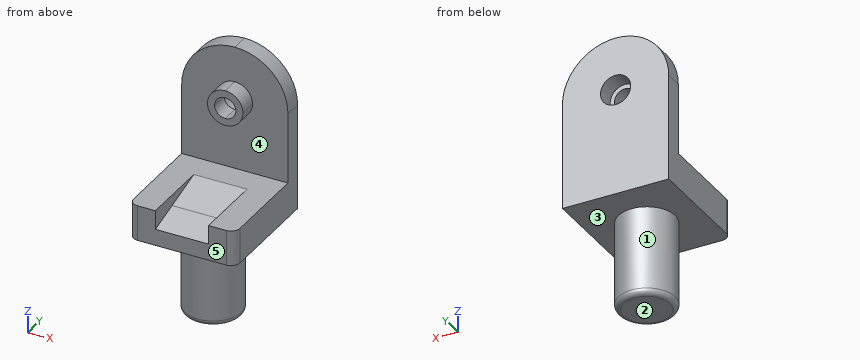
from build123d import *

# Parameters (mm, degrees)
F0_R      = 16
F1_DEPTH  = 50
F3_DEPTH  = 20
F4_DEPTH  = 20
F6_DEPTH  = 30
F7_DEPTH  = 40
F8_W      = 60
F8_H      = 10
F9_DEPTH  = 70
F10_R     = 29.99999
F11_R     = 3
F12_R     = 5
F14_D     = 17
F15_DEPTH = 10


# Not quite as in the source:
# - a fillet or chamfer is up to 0.001 mm smaller than in the source, because OpenCascade refuses the exact size


with BuildPart() as f1:
    # F0 (on Top) → F1 (new body)
    with BuildSketch(Plane.XY):
        Circle(F0_R)
    extrude(amount=F1_DEPTH)

    # F2 (on face) → F3 (join)
    with BuildSketch(Plane.XY.offset(50)):
        with BuildLine():
            Line((-30, 32.5), (-30, 7.5))
            Line((-30, 7.5), (-14.1332940251, 7.5))
            ThreePointArc((-14.1332940251, 7.5), (0, 16), (14.1332940251, 7.5))
            Line((14.1332940251, 7.5), (15, 7.5))
            Line((15, 7.5), (30, 7.5))
            Line((30, 7.5), (30, 32.5))
            Line((30, 32.5), (0, 32.5))
            Line((0, 32.5), (-30, 32.5))
        make_face()
        with BuildLine():
            ThreePointArc((14.1332940251, 7.5), (0, 16), (-14.1332940251, 7.5))
            Line((-14.1332940251, 7.5), (14.1332940251, 7.5))
        make_face()
    extrude(amount=F3_DEPTH)

    # F2 (on face) → F4 (join)
    with BuildSketch(Plane.XY.offset(50)):
        with BuildLine():
            Line((15, 5.5677643628), (15, -5.5677643628))
            ThreePointArc((15, -5.5677643628), (15.748015748, -2.8284271247), (16, 0))
            ThreePointArc((16, 0), (15.748015748, 2.8284271247), (15, 5.5677643628))
        make_face()
        with BuildLine():
            ThreePointArc((16, 0), (15.748015748, -2.8284271247), (15, -5.5677643628))
            Line((15, -5.5677643628), (15, -32.5))
            Line((15, -32.5), (30, -32.5))
            Line((30, -32.5), (30, 0))
            Line((30, 0), (30, 7.5))
            Line((30, 7.5), (15, 7.5))
            Line((15, 7.5), (15, 5.5677643628))
            ThreePointArc((15, 5.5677643628), (15.748015748, 2.8284271247), (16, 0))
        make_face()
    extrude(amount=F4_DEPTH)

    # F5 (on face) → F6 (join)
    with BuildSketch(Plane(origin=(15, 0, 0), x_dir=(0, -1, 0), z_dir=(-1, 0, 0))):
        Polygon((3.8423609018, 66.9608235561), (-7.5, 70), (-7.5, 50), (-5.5677643628, 50), (5.5677643628, 50), (32.5, 50), (32.5, 59.2820323028), (15.1847218036, 63.9216471122), align=None)
    extrude(amount=F6_DEPTH)

    # F7 (add): a face of the model
    f7_faces = [f1.faces().sort_by_distance(p)[0] for p in [
        (-22.5, 7.5, 60),
    ]]
    extrude(f7_faces, amount=F7_DEPTH)

    # F8 (on face) → F9 (join)
    with BuildSketch(Plane.XY.offset(70)):
        with Locations((0, 27.5)):
            Rectangle(F8_W, F8_H)
    extrude(amount=F9_DEPTH)

    # F10 (radius 30 in the source; OpenCascade refuses exactly that, so slightly less here)
    f10_edges = [f1.edges().sort_by_distance(p)[0] for p in [
        (-30, 27.5, 140),
        (30, 27.5, 140),
    ]]
    fillet(f10_edges, radius=F10_R)

    # F11
    f11_edges = [f1.edges().sort_by_distance(p)[0] for p in [
        (-16, 0, 0),
    ]]
    fillet(f11_edges, radius=F11_R)

    # F12
    f12_edges = [f1.edges().sort_by_distance(p)[0] for p in [
        (-30, -32.5, 60),
        (30, -32.5, 60),
    ]]
    fillet(f12_edges, radius=F12_R)

    # F14 (through all)
    with Locations(Plane.XZ.offset(-22.5)):
        with Locations((0, 110)):
            Hole(F14_D / 2)

    # F13 (on face) → F15 (join)
    with BuildSketch(Plane.XZ.offset(-22.5)):
        with BuildLine():
            Line((-6, 110), (-10, 110))
            ThreePointArc((-10, 110), (-7.0710678119, 102.9289321881), (0, 100))
            Line((0, 100), (0, 104))
            ThreePointArc((0, 104), (-4.2426406871, 105.7573593129), (-6, 110))
        make_face()
        with BuildLine():
            Line((0, 116), (0, 120))
            ThreePointArc((0, 120), (-7.0710678119, 117.0710678119), (-10, 110))
            Line((-10, 110), (-6, 110))
            ThreePointArc((-6, 110), (-4.2426406871, 114.2426406871), (0, 116))
        make_face()
        with BuildLine():
            ThreePointArc((10, 110), (7.0710678119, 117.0710678119), (0, 120))
            Line((0, 120), (0, 116))
            ThreePointArc((0, 116), (4.2426406871, 114.2426406871), (6, 110))
            Line((6, 110), (10, 110))
        make_face()
        with BuildLine():
            ThreePointArc((0, 100), (7.0710678119, 102.9289321881), (10, 110))
            Line((10, 110), (6, 110))
            ThreePointArc((6, 110), (4.2426406871, 105.7573593129), (0, 104))
            Line((0, 104), (0, 100))
        make_face()
    extrude(amount=F15_DEPTH)


solid = f1.part
Input: part model. Units: mm. Frame: model coordinates. Face numbers are marked on the shaded views. A direction names the side the tool comes from. Round coordinates to 2 decimals unless told otherwise and drop trailing zeros. Loops run counter-clockwise (first coordinate to the right, second up) from the corner with the lowest first, then second, coordinate; pieces in that order, holes last. Notation, with made-up numbers: (72, -31.75) -> (83, -31.75) arc R19 cw to (83, -20.75) -> close; hole circle Ø5 at (20.5, -0.5). An arc over 180 degrees is marked (long way). Answer as a JSON object with one key per item and string values. Group by question number.
1) Pin query (flat end, axial travel): pin 1 (13.5 mm diameter, centred on x = -0.5, z = 111.5, fed in from +Y); pin 2 (22 mm diameter, centred on x = 0, z = 110, fed in from +Y); pin 3 (12 mm diameter, centred on x = 6, z = 114.5, fed in from -Y); pin 4 (3 mm diameter, centred on x = 14, y = 8.5, fed in from -Z). Return the tip coordinate at first contact, or that it passes through.
2) Ray query, L1, parallel to Z at x = 0.5, y = 29; L2, parallel to Y at x = -15, z = 108; L3, parallel to Z at x = 19.5, y = 3.5. Return the intervals inside material, ascending.
3) Section query B-B on y = 14.5. State how many separate pieces and enclosed holes the cut face has, plus the area to 3 significant figures.
4) Section query D-D on y = 0. Output: boundary loops of the cut face in (x, z).
5) Section query C-C on x = -20.5. Output: boundary loops of the cut face in (y, z).
6) Reachability of the marked faces 1 and 2 from +Z, -Z, +X, -X, +Y, -Y: full face, straight path, thin tool, end or side. Return the list, or none.
7) Section query A-A on z = 106.5. Output: boundary loops of the cut face in (x, y), plus the area to 3 significant figures.
8) Draft query along Z for the marked faces 3, 4 and 5. Return one class per face: +Z half, -Z half, draft (parallel to the pull), parting line (faces both ways), or undercut.
Reply:
{
 "1": {"pin 1": "stops at y = 22.5", "pin 2": "stops at y = 32.5", "pin 3": "stops at y = 12.5", "pin 4": "stops at z = 0.66"},
 "2": {"L1": "z = 50 to 101.51, 118.49 to 140", "L2": "y = 22.5 to 32.5", "L3": "z = 50 to 70"},
 "3": {"separate pieces": "2", "enclosed holes": "1", "area": "2,070 mm2"},
 "4": {"outline": "(-30, 50) -> (-16, 50) -> (-16, 3) arc R3 ccw to (-13, 0) -> (13, 0) arc R3 ccw to (16, 3) -> (16, 50) -> (30, 50) -> (30, 70) -> (15, 70) -> (15, 67.99) -> (-15, 67.99) -> (-15, 70) -> (-30, 70) -> close"},
 "5": {"outline": "(-32.5, 50) -> (32.5, 50) -> (32.5, 131.9) -> (22.5, 131.9) -> (22.5, 70) -> (-32.5, 70) -> close"},
 "6": {"face 1": "-Z", "face 2": "-Z, +X, -X, +Y, -Y"},
 "7": {"outline": "(-30, 22.5) -> (-9.37, 22.5) -> (-9.37, 12.5) -> (-4.87, 12.5) -> (-4.87, 22.5) -> (-7.75, 22.5) -> (-7.75, 32.5) -> (-30, 32.5) -> close; (4.87, 12.5) -> (9.37, 12.5) -> (9.37, 22.5) -> (30, 22.5) -> (30, 32.5) -> (7.75, 32.5) -> (7.75, 22.5) -> (4.87, 22.5) -> close", "area": "535 mm2"},
 "8": {"face 3": "-Z half", "face 4": "undercut", "face 5": "draft"}
}
